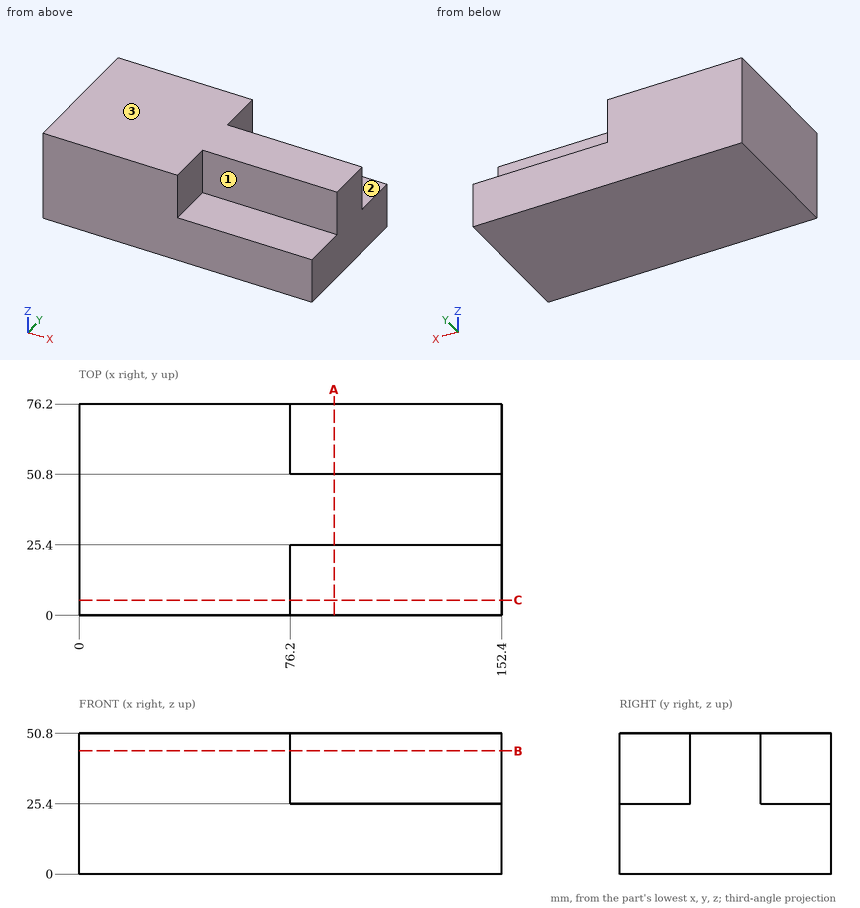
Part print with two shaded views. Sizes in mm from the minimum x, y, z corner. A direction names the side the tool comes from. Give positions to 0.01 mm unless a question says otherwise; leave off trailing zeros. Order: outer loops, then holes, each group sorted by start corner. A loop starts at its lowest first (then second) coordinate and runs counter-clockwise, first axis right, second up.
1) Saw through at C-C, the plane y = 5.5. Write the cut outline in (x, z).
2) Pin check, flat tips, straight feed: pin 1 (12.5 mm diameter, centred on x = 96, z = 33.5, fed in from -Y); pin 2 (12.5 mm diameter, centred on y = 65, z = 38.5, fed in from +X); pin 3 (7.5 mm diameter, centred on x = 127.5, y = 67.5, fed in from +Z). Stop position of each tip, or through.
3) Saw through at B-B, the plane z = 44.5. Write the cut outline in (x, y), then the cut area to 3 significant figures.
4) Wall check: probe 1 along X at (y, z) = (16, 32); probe 2 along Y at (x, z) = (94, 32); probe 3 along Z at (x, y) = (82, 14). Give the ranges that are in metal, low to high.
5) Saw through at A-A, the plane x = 92. Write the cut outline in (y, z), then the cut area to 3 significant figures.
6) 3-axis set-ups, long thin cutter, end or side, ignore diameter. For the marked faces 1, 2 and 3: which of +Z, -Z, +X, -X, +Y, -Y reach the whole face in a straight line?
Computed:
1. outline: (0, 0) - (152.4, 0) - (152.4, 25.4) - (76.2, 25.4) - (76.2, 50.8) - (0, 50.8) - close
2. pin 1: stops at y = 25.4
2. pin 2: stops at x = 76.2
2. pin 3: stops at z = 25.4
3. outline: (0, 0) - (76.2, 0) - (76.2, 25.4) - (152.4, 25.4) - (152.4, 50.8) - (76.2, 50.8) - (76.2, 76.2) - (0, 76.2) - close
3. area: 7,740 mm2
4. probe 1: x = 0 to 76.2
4. probe 2: y = 25.4 to 50.8
4. probe 3: z = 0 to 25.4
5. outline: (0, 0) - (76.2, 0) - (76.2, 25.4) - (50.8, 25.4) - (50.8, 50.8) - (25.4, 50.8) - (25.4, 25.4) - (0, 25.4) - close
5. area: 2,580 mm2
6. face 1: +Z, +X, -Y
6. face 2: +Z, +X, +Y
6. face 3: +Z, +X, -X, +Y, -Y
